Work out the finished part from the listing and answer in its coordinate system (mm). Face numbers are marked on the shaded views. A direction names the side the tool comes from. Give positions to 0.01 mm unless a question says otherwise; leave off trailing zeros. Loops run counter-clockwise (first coordinate to the right, second up) from the corner with the lowest first, then second, coordinate; pieces in that order, holes last.
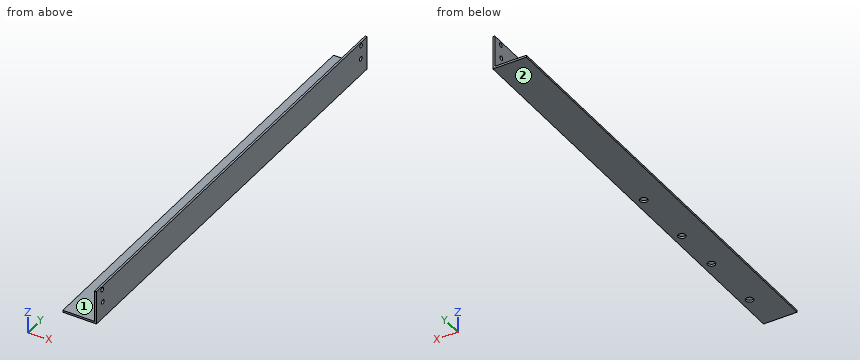
Autodesk Inventor part; units mm, degrees
ref_plane "YZ Plane" through (0, 0, 0) normal (1, 0, 0) x (0, 1, 0)
ref_plane "XZ Plane" through (0, 0, 0) normal (0, 1, 0) x (-1, 0, 0)
ref_plane "XY Plane" through (0, 0, 0) normal (0, 0, 1) x (1, 0, 0)
sketch "Sketch1" plane through (0, 0, 0) normal (0, 1, 0) x (-1, 0, 0)
  line L0 (0, 0) -> (50, 0)
  line L1 (50, 0) -> (50, 3)
  line L2 (0, 0) -> (0, 50)
  line L3 (0, 50) -> (3, 50)
  line L4 (3, 50) -> (3, 3)
  line L5 (3, 3) -> (50, 3)
  dimension "d0" = 50
  dimension "d1" = 3
  dimension "d2" = 50
  dimension "d3" = 3
extrude "Extrusion1" add sketch "Sketch1" along normal blind 660.4
sketch "Sketch3" plane through (0, 0, 50) normal (1, 0, 0) x (0, 0, -1)
  circle A0 centre (25, 15.7) radius 3.175
  circle A1 centre (25, 644.7) radius 3.175
  dimension "d57" = 6.35
  dimension "d59" = 6.35
extrude "Extrusion3" cut sketch "Sketch3" against normal blind 25.4
sketch "Sketch4" plane through (0, 0, 50) normal (1, 0, 0) x (0, 0, -1)
  circle A0 centre (5.3, 645.6513) radius 3.175
extrude "Extrusion4" cut sketch "Sketch4" against normal blind 25.4
sketch "Sketch5" plane through (0, 0, 50) normal (1, 0, 0) x (0, 0, -1)
  circle A0 centre (5.3, 13.8784) radius 3.175
extrude "Extrusion5" cut sketch "Sketch5" against normal blind 25.4
sketch "Sketch6" plane through (0, 0, 0) normal (0, 0, -1) x (-1, 0, 0)
  circle A0 centre (12.7942, 55.1) radius 5.5
  circle A1 centre (12.7942, 148.1) radius 5.5
  circle A2 centre (12.7942, 220.2) radius 5.5
  circle A3 centre (12.7942, 313.2) radius 5.5
extrude "Extrusion6" cut sketch "Sketch6" against normal blind 25.4
equation "\"d59\" = d57"
properties part number "26in Angle Channel CIM Mount Right" material "Aluminum 6061"
Q1. Section A-A on y = 148.1 is taken. Give the vertices of the cut face in (x, z).
Q2. Section B-B on x = -29 is taken. Give the vertices of the cut face in (y, z).
Q3. Which of the six approach directions +Z, -Z, +X, -X, +Y, -Y give full straight-line access (tool end or side, diameter ignored) to the marked faces 1 and 2?
Q4. Given pin 1 (14.5 mm diameter, centred on x = -12.79, y = 55.1, fed in from +Z); pin 2 (8.5 mm diameter, centred on y = 644.7, z = 25, fed in from +X); pin 3 (5 mm diameter, centred on y = 645.65, z = 44.7, fed in from +X); pin 4 (10 mm diameter, centred on y = 187.5, z = 21.5, fed in from -X), each flat-ended and moving along its own axis, determine where each tip first touches the part or whether it passes through.
Q5. Consider line 1 along Y through (x, z) = (-1.05, 44.7); line 2 along X through (y, z) = (313.2, 2.05); line 3 along X through (y, z) = (138, 9). Determine where each line is inside the solid, lowest interval first.
Check result:
1. outline: (-50, 0) - (-18.29, 0) - (-18.29, 3) - (-50, 3) - close; (-7.29, 0) - (0, 0) - (0, 50) - (-3, 50) - (-3, 3) - (-7.29, 3) - close
2. outline: (0, 0) - (660.4, 0) - (660.4, 3) - (0, 3) - close
3. face 1: +Z, -X, +Y, -Y
3. face 2: -Z, +X, -X, +Y, -Y
4. pin 1: stops at z = 3
4. pin 2: stops at x = 0
4. pin 3: passes through
4. pin 4: stops at x = -3
5. line 1: y = 0 to 10.7, 17.05 to 642.48, 648.83 to 660.4
5. line 2: x = -50 to -18.29, -7.29 to 0
5. line 3: x = -3 to 0
